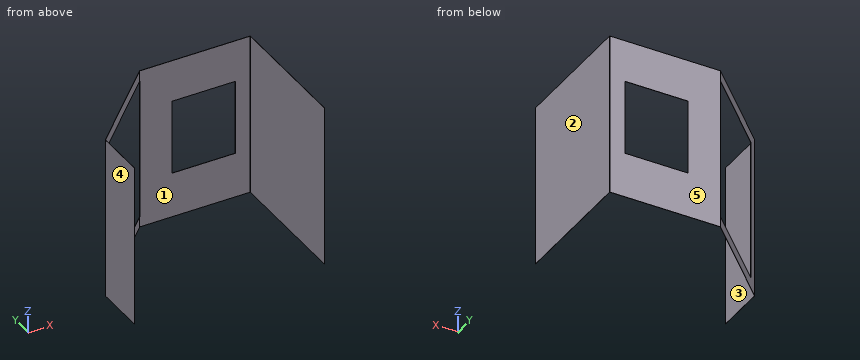
```python
from build123d import *

# Parameters (mm, degrees)
SALIENTE_EXTRUIR1_DEPTH    = 0.83566
SALIENTE_EXTRUIR2_DEPTH    = 12.7
SALIENTE_EXTRUIR3_DEPTH    = 642.126
CROQUIS4_W                 = 255
CROQUIS4_H                 = 0.83566
SALIENTE_EXTRUIR4_DEPTH    = 170
CROQUIS5_W                 = 255
CROQUIS5_H                 = 0.83566
SALIENTE_EXTRUIR5_DEPTH    = 170
CROQUIS6_W                 = 570
CROQUIS6_H                 = 401.24062337
CORTAR_EXTRUIR1_DEPTH      = 190
CORTAR_EXTRUIR2_DEPTH      = 198
CORTAR_EXTRUIR2_DEPTH_BACK = 174
REDONDEO3_R                = 0.8


with BuildPart() as part:
    # Croquis1 → Saliente-Extruir1 (new body)
    with BuildSketch(Plane.XY):
        Polygon((0, 0), (765, 0), (765, 525), (320, 525), (0, 205), align=None)
    extrude(amount=SALIENTE_EXTRUIR1_DEPTH)

    # Croquis7 → Cortar-Extruir2 (cut, two sides: drawn at the far end of the back side and taken through both)
    with BuildSketch(Plane.XY.offset(0.83566).offset(-CORTAR_EXTRUIR2_DEPTH_BACK)):
        Polygon((0, 0), (765, 0), (765, 525), (320, 525), (0, 205), align=None)
    extrude(amount=CORTAR_EXTRUIR2_DEPTH + CORTAR_EXTRUIR2_DEPTH_BACK, mode=Mode.SUBTRACT)


with BuildPart() as body_2:
    # Croquis2 → Saliente-Extruir2 (new body)
    with BuildSketch(Plane.XY.offset(0.83566)):
        Polygon((765.83566, 525.83566), (319.653858294, 525.83566), (-0.83566, 205.346141706), (-0.83566, 0), (0, 0), (0, 205), (320, 525), (765, 525), (765, 0), (765.83566, 0), align=None)
    extrude(amount=SALIENTE_EXTRUIR2_DEPTH)

    # Croquis3 → Saliente-Extruir3 (add)
    with BuildSketch(Plane.XY.offset(13.53566)):
        Polygon((450, 525.83566), (450, 525), (320, 525), (0, 205), (0, 0), (-0.83566, 0), (-0.83566, 205.346141706), (319.653858294, 525.83566), align=None)
        Polygon((765.83566, 0), (765.83566, 525.83566), (705, 525.83566), (705, 525), (765, 525), (765, 0), align=None)
    extrude(amount=SALIENTE_EXTRUIR3_DEPTH)

    # Croquis4 → Saliente-Extruir4 (add)
    with BuildSketch(Plane.XY.offset(13.53566)):
        with Locations((577.5, 525.41783)):
            Rectangle(CROQUIS4_W, CROQUIS4_H)
    extrude(amount=SALIENTE_EXTRUIR4_DEPTH)

    # Croquis5 → Saliente-Extruir5 (add)
    with BuildSketch(Plane.XY.offset(655.66166)):
        with Locations((577.5, 525.41783)):
            Rectangle(CROQUIS5_W, CROQUIS5_H)
    extrude(amount=-SALIENTE_EXTRUIR5_DEPTH)

    # Croquis6 → Cortar-Extruir1 (cut)
    with BuildSketch(Plane(origin=(-103.090900853, 103.090900853, 0), x_dir=(0, 0, 1), z_dir=(-0.7071067811865477, 0.7071067811865475, 0))):
        with Locations((328.24866, 397.231060123)):
            Rectangle(CROQUIS6_W, CROQUIS6_H)
    extrude(amount=-CORTAR_EXTRUIR1_DEPTH, mode=Mode.SUBTRACT)

    # Redondeo3
    redondeo3_edges = [body_2.edges().sort_by_distance(p)[0] for p in [
        (0, 205, 328.24866),
        (-0.83566, 205.346141706, 328.24866),
        (765.83566, 525.83566, 328.24866),
        (765, 525, 328.24866),
    ]]
    fillet(redondeo3_edges, radius=REDONDEO3_R)


solid = body_2.part
```
Geometry check sheet. Reference: the model listing, model coordinates, mm. Face numbers are marked on the shaded views. A direction names the side the tool comes from. Give positions to 0.01 mm unless a question says otherwise; leave off trailing zeros. Write each loop counter-clockwise with the first axis right and the second up, starting at its lowest first coordinate (ties: lowest second). Pieces come first, ordered by that corner, then holes.
1) Release check for a two-part mould opening along X. For the marked faces 3, 4 and 5 record: pulls with the +X half, pulls with the -X half, needs draft (parallel to the pull), parting line crosses it, or undercut.
2) Section check B-B, the plane z = 217.5. Record the boundary of the cut face in (x, y), and give its area (3 significant figures).
3) Access from +Z, -Z, +X, -X, +Y, -Y to the whole of each face (thin tool, end or side, straight path). Record for the marked faces 1 and 2.
4) Section check D-D, the plane z = 551.5. Record the boundary of the cut face in (x, y), and give its area (3 significant figures).
5) Section check A-A, the plane x = 474.5. Record the boundary of the cut face in (y, z), and give its area (3 significant figures).
6) Gauge pin test, flat ends, axial feed: pin 1 (0.9 mm diameter, centred on y = 525, z = 274.5, fed in from -X); pin 2 (1 mm diameter, centred on y = 237, z = 246.5, fed in from -X); pin 3 (1 mm diameter, centred on x = 354.5, z = 178, fed in from -Y). Record the tip position at first contact, or that the pin passes through.
7) Section check C-C, the plane y = 76. Record the boundary of the cut face in (x, z), and give its area (3 significant figures).
8) Material ranges on L1, parallel to X at y = 180, z = 473; L2, parallel to Y at x = 409, z = 269.5; L3, parallel to X at y = 322.5, z = 32.5, recorded low to high.
Computed:
1. face 3: undercut
1. face 4: pulls with the -X half
1. face 5: needs draft
2. outline: (-0.84, 0) - (0, 0) - (0, 204.67) arc R0.8 cw to (0.23, 205.23) - (36.52, 241.52) - (35.93, 242.12) - (-0.6, 205.58) arc R0.8 ccw to (-0.84, 205.01) - close; (319.65, 525.84) - (320.49, 525) - (450, 525) - (450, 525.84) - close; (705, 525) - (764.2, 525) arc R0.8 cw to (765, 524.2) - (765, 0) - (765.84, 0) - (765.84, 525.04) arc R0.8 ccw to (765.04, 525.84) - (705, 525.84) - close
2. area: 813 mm2
3. face 1: +Z, -Z, -Y
3. face 2: +Z, -Z, +X, +Y, -Y
4. outline: (-0.84, 0) - (0, 0) - (0, 204.67) arc R0.8 cw to (0.23, 205.23) - (36.52, 241.52) - (35.93, 242.12) - (-0.6, 205.58) arc R0.8 ccw to (-0.84, 205.01) - close; (319.65, 525.84) - (320.49, 525) - (764.2, 525) arc R0.8 cw to (765, 524.2) - (765, 0) - (765.84, 0) - (765.84, 525.04) arc R0.8 ccw to (765.04, 525.84) - close
4. area: 1,030 mm2
5. outline: (525, 0.84) - (525.84, 0.84) - (525.84, 183.54) - (525, 183.54) - close; (525, 485.66) - (525.84, 485.66) - (525.84, 655.66) - (525, 655.66) - close
5. area: 295 mm2
6. pin 1: stops at x = 320.04
6. pin 2: stops at x = 30.32
6. pin 3: stops at y = 525
7. outline: (-0.84, 0.84) - (0, 0.84) - (0, 655.66) - (-0.84, 655.66) - close; (765, 0.84) - (765.84, 0.84) - (765.84, 655.66) - (765, 655.66) - close
7. area: 1,090 mm2
8. L1: x = -0.84 to 0, 765 to 765.84
8. L2: y = 525 to 525.84
8. L3: x = 116.32 to 117.5, 765 to 765.84
